For this review, take the finished solid that the model builds, in its own axes (mm). A direction names the side the tool comes from. Give positions to 0.01 mm unless a question says otherwise; leave off trailing zeros. Order: outer loops, then holes, each group sorted by start corner. A loop starts at its lowest first (then second) coordinate and runs counter-clockwise, first axis right, second up. Notation, with made-up numbers: M 49.25,83 L 102.25,83 A18 ccw 102.25,89 Z; hole C -8.5,88 d2. An arc over 180 degrees is marked long. Use CSV: the item, a comma, the result in double quotes. Start each with the question number.
(1) Consider section C-C (z = 2.25). Write out the cut boundary in (x, y), and give its area (3 significant figures).
(2) Consider section D-D (y = 4.75). Write out the cut boundary in (x, z).
(3) Consider section A-A (x = 0). Write out the cut boundary in (y, z) (3 decimals).
(4) Wall thickness on L1, parallel to Z at x = 0, y = 7.1 (3 decimals); L2, parallel to X at y = 6.5, z = -1.5: over which ranges is each line inside the solid? List them lowest first. Write a range as from..to.
(5) Draft analysis for pull direction Z (two halves, no side actions). For faces 4 (the face through (-0.69, 7.64, 3.1)), 5 (the face through (-3, 0, 0)), 6 (the face through (-0.661, 4.383, -5.037)), state which applies: pulls with the +Z half, pulls with the -Z half, needs draft (parallel to the pull), parting line crosses it, or undercut.
(6) Consider section B-B (y = 7.5). Write out the cut boundary in (x, z) (3 decimals), and give its area (3 significant figures).
(7) Clearance check with flat-ended pins moving along their axes: P1, Ø2, axis at x = 3, y = 2, coming from the -Z side; P2, Ø4, axis at y = 3.5, z = 2.5, coming from the -X side; P3, Ø1.9, axis at x = 1, z = -0.5, coming from the -Y side. State where each tip first meets the part, or that it passes through.
(8) Tool access review of faces 1 (the face through (0, 3.81, 0)), 2 (the face through (3.3, 8.89, 1.1)), 3 (the face through (0, 6.35, 0)): name each direction out of +Z, -Z, +X, -X, +Y, -Y from which nothing blocks a thin tool from reaching the whole face with its end or side.
```python
from build123d import *

# Parameters (mm, degrees)
SKETCH1_R           = 5.08
BOSS_EXTRUDE1_DEPTH = 8.89
CUT_EXTRUDE1_DEPTH  = 3.81
SKETCH3_R           = 3.175
CUT_EXTRUDE2_DEPTH  = 2.54


with BuildPart() as part:
    # Sketch1 → Boss-Extrude1 (new body)
    with BuildSketch(Plane(origin=(0, 0, 0), x_dir=(1, 0, 0), z_dir=(0, 1, 0))):
        Circle(SKETCH1_R)
    extrude(amount=BOSS_EXTRUDE1_DEPTH)

    # Sketch2 → Cut-Extrude1 (cut)
    with BuildSketch(Plane(origin=(0, 0, 0), x_dir=(1, 0, 0), z_dir=(0, 1, 0))):
        with BuildLine():
            Line((-2.794, 1.987864432), (-2.794, -1.987864432))
            ThreePointArc((-2.794, -1.987864432), (1.043411472, -3.266394572), (3.429, 0))
            ThreePointArc((3.429, 0), (1.043411472, 3.266394572), (-2.794, 1.987864432))
        make_face()
    extrude(amount=CUT_EXTRUDE1_DEPTH, mode=Mode.SUBTRACT)

    # Sketch3 → Cut-Extrude2 (cut)
    with BuildSketch(Plane(origin=(0, 8.89, 0), x_dir=(1, 0, 0), z_dir=(0, 1, 0))):
        Circle(SKETCH3_R)
    extrude(amount=-CUT_EXTRUDE2_DEPTH, mode=Mode.SUBTRACT)


solid = part.part
```
Check result:
1,outline,"M -4.55,0 L -2.59,0 L -2.59,3.81 L 2.59,3.81 L 2.59,0 L 4.55,0 L 4.55,8.89 L 2.24,8.89 L 2.24,6.35 L -2.24,6.35 L -2.24,8.89 L -4.55,8.89 Z"
1,area,"49.9 mm^2"
2,outline,"C 0,0 d10.16"
3,outline,"M 0,-5.08 L 8.89,-5.08 L 8.89,-3.175 L 6.35,-3.175 L 6.35,3.175 L 8.89,3.175 L 8.89,5.08 L 0,5.08 L 0,3.429 L 3.81,3.429 L 3.81,-3.429 L 0,-3.429 Z"
4,L1,"z = -5.08..-3.175, 3.175..5.08"
4,L2,"x = -4.85..-2.8, 2.8..4.85"
5,face 4,"undercut"
5,face 5,"needs draft"
5,face 6,"parting line crosses it"
6,outline,"C 0,0 d10.16; hole C 0,0 d6.35"
6,area,"49.4 mm^2"
7,P1,"stops at z = -4.67"
7,P2,"stops at x = -5.06"
7,P3,"stops at y = 3.81"
8,face 1,"-Y"
8,face 2,"+Z, -Z, +X, -X, +Y"
8,face 3,"+Y"
